```python
from build123d import *

# Parameters (mm, degrees)
F3_DEPTH = 60.001


with BuildPart() as f1:
    # F0 (on Front) → F1 (revolve)
    with BuildSketch(Plane.XZ):
        Polygon((40, 30), (25, 30), (25, -30), (40, -30), (50, -30), (60, -30), (60, -25), (50, -20), (50, -10), (60, -5), (60, 5), (50, 10.338278207), (50, 20), (60, 25), (60, 30), (50, 30), align=None)
    revolve(axis=Axis((0, 0, 0), (0, 0, -1)))

    # F2 (on face) → F3 (cut, through all)
    with BuildSketch(Plane.XY.offset(30)):
        with BuildLine():
            Line((7.5, 31), (-7.5, 31))
            Line((-7.5, 31), (-7.5, 23.8484800354))
            ThreePointArc((-7.5, 23.8484800354), (0, 25), (7.5, 23.8484800354))
            Line((7.5, 23.8484800354), (7.5, 31))
        make_face()
    extrude(amount=-F3_DEPTH, mode=Mode.SUBTRACT)


solid = f1.part
```
The model under review builds one solid part; all positions refer to its coordinate system, in mm. A direction names the side the tool comes from. Round coordinates to 2 decimals unless told otherwise and drop trailing zeros. Order: outer loops, then holes, each group sorted by start corner. A loop starts at its lowest first (then second) coordinate and runs counter-clockwise, first axis right, second up. Notation, with made-up numbers: (-27, -27) - (-21, -27) arc R10 ccw to (-21, -13) - close; hole circle Ø10 at (4, 72). An arc over 180 degrees is marked (long way). Answer in a Markdown table with one row per item.
(1) Take a section at B-B on y = 0. Write out the cut boundary in (x, z), plus the area to 3 significant figures.
Result set:
| item | result |
|---|---|
| outline | (-60, -30) - (-25, -30) - (-25, 30) - (-60, 30) - (-60, 25) - (-50, 20) - (-50, 10.34) - (-60, 5) - (-60, -5) - (-50, -10) - (-50, -20) - (-60, -25) - close; (25, -30) - (60, -30) - (60, -25) - (50, -20) - (50, -10) - (60, -5) - (60, 5) - (50, 10.34) - (50, 20) - (60, 25) - (60, 30) - (25, 30) - close |
| area | 3,600 mm2 |
(2) Take a section at D-D on z = 7. Write out the cut boundary in (x, y), plus the area to 3 significant figures.
Result set:
| item | result |
|---|---|
| outline | circle Ø112.51 at (0, 0); hole (-7.5, 23.85) arc R25 ccw (long way) to (7.5, 23.85) - (7.5, 31) - (-7.5, 31) - close |
| area | 7,880 mm2 |
(3) Mouldability with a two-part tool opening along Y and no side actions: class faces 1 (the face through (-26, -1, -30)), 2 (the face through (-59.94, -2.64, -27.46)), 3 (the face through (7.5, 27, 0)) as released by +Y, released by -Y, zero draft, split by the parting line, or undercut.
Result set:
| item | result |
|---|---|
| face 1 | zero draft |
| face 2 | split by the parting line |
| face 3 | undercut |
(4) Take a section at C-C on z = 0. Write out the cut boundary in (x, y).
Result set:
| item | result |
|---|---|
| outline | circle Ø120 at (0, 0); hole (-7.5, 23.85) arc R25 ccw (long way) to (7.5, 23.85) - (7.5, 31) - (-7.5, 31) - close |
(5) Clearance check with flat-ended pins moving along their axes: P1, Ø3.5, axis at y = 29, z = 4.5, coming from the +X side (3 decimals); P2, Ø1.5, axis at y = 28.5, z = 17.5, coming from the +X side; P3, Ø5, axis at x = 45.5, z = 3, coming from the +Y side. State where each tip first meets the part, or that it passes through.
Result set:
| item | result |
|---|---|
| P1 | stops at x = 53.455 |
| P2 | stops at x = 41.59 |
| P3 | stops at y = 41.84 |
(6) Take a section at A-A on x = 0. Write out the cut boundary in (y, z), plus the area to 3 significant figures.
Result set:
| item | result |
|---|---|
| outline | (-60, -30) - (-25, -30) - (-25, 30) - (-60, 30) - (-60, 25) - (-50, 20) - (-50, 10.34) - (-60, 5) - (-60, -5) - (-50, -10) - (-50, -20) - (-60, -25) - close; (31, -30) - (60, -30) - (60, -25) - (50, -20) - (50, -10) - (60, -5) - (60, 5) - (50, 10.34) - (50, 20) - (60, 25) - (60, 30) - (31, 30) - close |
| area | 3,240 mm2 |
(7) For line 1 (X direction, y = 0, z = -16); line 2 (Z direction, x = -45, y = 34); line 3 (Y direction, x = 0, z = 16.5), list the stretches that pass through material, from the lowest coordinate up. Write a range as from..to.
Result set:
| item | result |
|---|---|
| line 1 | x = -50..-25, 25..50 |
| line 2 | z = -30..-23.2, -6.8..6.92, 23.2..30 |
| line 3 | y = -50..-25, 31..50 |
(8) Machinability: for faces 4 (the face through (-7.5, 27, 0)), 5 (the face through (27.216, -42.688, -9.687)), 6 (the face through (26, -1, 30)), which of the approach directions +Z, -Z, +X, -X, +Y, -Y give a long, thin tool a straight path to every point of the face, cutting with its end or side? Answer none if there is none.
Result set:
| item | result |
|---|---|
| face 4 | +Z, -Z |
| face 5 | none |
| face 6 | +Z, +X, -X, +Y, -Y |
